Geometry: final body of the model. Coordinates: model frame, mm. A direction names the side the tool comes from. Round coordinates to 2 decimals unless told otherwise and drop trailing zeros. Order: outer loops, then holes, each group sorted by start corner. A loop starts at its lowest first (then second) coordinate and runs counter-clockwise, first axis right, second up. Notation, with made-up numbers: (20, 19) - (32, 19) arc R9 cw to (32, 36) - close; hole circle Ø7 at (2.25, 20). An arc over 180 degrees is marked (long way). Put each result on its own line as item: value. Start each with the question number.
(1) Access query for faces 3 (the face through (22.121, 0.986, -7.114)), 4 (the face through (-17.948, 0.986, 9.927)), 5 (the face through (5.273, 0.986, 18.594)). Directions: +Z, -Z, +X, -X, +Y, -Y. A direction counts if a zero-diameter tool reaches every point of the face in a straight line with its end or side. Return the directions, or none.
(2) Pull-direction query (Z, two-part tool) for faces 1 (the face through (22.596, 0.986, -2.222)), 2 (the face through (17.22, 0.99, 15.6)); classes: released by +Z, released by -Z, zero draft, split by the parting line, or undercut.
(3) Section A-A (x = 0). Output: boundary loops of the cut face in (y, z), and give its area (3 significant figures).
(4) Pin query (flat end, axial travel): P1, Ø0.6, axis at x = -5, y = 1, coming from the +Z side; P2, Ø1, axis at x = 4, y = 1, coming from the -Z side; P3, Ø0.6, axis at y = 1, z = 5.5, coming from the +X side. Return the tip coordinate at first contact, or that it passes through.
(5) Section B-B (z = 0). Output: boundary loops of the cut face in (x, y), and give its area (3 significant figures).
(6) Material intervals for L1, parallel to X at y = 0.45, z = 7.5; L2, parallel to X at y = 1.75, z = -21; L3, parallel to Z at x = 5.5, y = 1.35, sorted ascending. Write a range as [from, to].
(7) Section C-C (y = 0.45). Count the separate pieces of the cut face and the enclosed holes in it, and give its area (3 significant figures).
from build123d import *

# Parameters (mm, degrees)
SKETCH_1_R      = 1
SKETCH_1_R_2    = 12.835097572
EXTRUDE_1_DEPTH = 2


with BuildPart() as part:
    # 草图1 → 凸台-拉伸1 (new body)
    with BuildSketch(Plane(origin=(0, 0, 0), x_dir=(1, 0, 0), z_dir=(0, 1, 0))):
        with BuildLine():
            Line((7.150459564, 22.71458211), (2.584896164, 22.71458211))
            Line((2.584896164, 22.71458211), (-1.893440977, 18.236244969))
            Line((-1.893440977, 18.236244969), (-6.310791907, 15.68588622))
            ThreePointArc((-6.310791907, 15.68588622), (-7.676817311, 16.051911624), (-7.310791907, 17.417937028))
            Line((-7.310791907, 17.417937028), (-3.177406319, 19.80434831))
            ThreePointArc((-3.177406319, 19.80434831), (-2.244981501, 22.637541774), (-5.164811424, 23.246634926))
            Line((-5.164811424, 23.246634926), (-9.118705311, 20.963853226))
            Line((-9.118705311, 20.963853226), (-10.757890471, 14.846330924))
            Line((-10.757890471, 14.846330924), (-13.30824922, 10.428979994))
            ThreePointArc((-13.30824922, 10.428979994), (-14.674274623, 10.06295459), (-15.040300027, 11.428979994))
            Line((-15.040300027, 11.428979994), (-12.653888745, 15.562365582))
            ThreePointArc((-12.653888745, 15.562365582), (-13.262981897, 18.482195505), (-16.096175362, 17.549770686))
            Line((-16.096175362, 17.549770686), (-18.378957062, 13.5958768))
            Line((-18.378957062, 13.5958768), (-16.739771901, 7.478354497))
            Line((-16.739771901, 7.478354497), (-16.739771901, 2.377637001))
            ThreePointArc((-16.739771901, 2.377637001), (-17.739771901, 1.377637001), (-18.739771901, 2.377637001))
            Line((-18.739771901, 2.377637001), (-18.739771901, 7.150459564))
            ThreePointArc((-18.739771901, 7.150459564), (-20.727177006, 9.374559877), (-22.71458211, 7.150459564))
            Line((-22.71458211, 7.150459564), (-22.71458211, 2.584896164))
            Line((-22.71458211, 2.584896164), (-18.236244969, -1.893440977))
            Line((-18.236244969, -1.893440977), (-15.68588622, -6.310791907))
            ThreePointArc((-15.68588622, -6.310791907), (-16.051911624, -7.676817311), (-17.417937028, -7.310791907))
            Line((-17.417937028, -7.310791907), (-19.80434831, -3.177406319))
            ThreePointArc((-19.80434831, -3.177406319), (-22.637541774, -2.244981501), (-23.246634926, -5.164811424))
            Line((-23.246634926, -5.164811424), (-20.963853226, -9.118705311))
            Line((-20.963853226, -9.118705311), (-14.846330924, -10.757890471))
            Line((-14.846330924, -10.757890471), (-10.428979994, -13.30824922))
            ThreePointArc((-10.428979994, -13.30824922), (-10.06295459, -14.674274623), (-11.428979994, -15.040300027))
            Line((-11.428979994, -15.040300027), (-15.562365582, -12.653888745))
            ThreePointArc((-15.562365582, -12.653888745), (-18.482195505, -13.262981897), (-17.549770686, -16.096175362))
            Line((-17.549770686, -16.096175362), (-13.5958768, -18.378957062))
            Line((-13.5958768, -18.378957062), (-7.478354497, -16.739771901))
            Line((-7.478354497, -16.739771901), (-2.377637001, -16.739771901))
            ThreePointArc((-2.377637001, -16.739771901), (-1.377637001, -17.739771901), (-2.377637001, -18.739771901))
            Line((-2.377637001, -18.739771901), (-7.150459564, -18.739771901))
            ThreePointArc((-7.150459564, -18.739771901), (-9.374559877, -20.727177006), (-7.150459564, -22.71458211))
            Line((-7.150459564, -22.71458211), (-2.584896164, -22.71458211))
            Line((-2.584896164, -22.71458211), (1.893440977, -18.236244969))
            Line((1.893440977, -18.236244969), (6.310791907, -15.68588622))
            ThreePointArc((6.310791907, -15.68588622), (7.676817311, -16.051911624), (7.310791907, -17.417937028))
            Line((7.310791907, -17.417937028), (3.177406319, -19.80434831))
            ThreePointArc((3.177406319, -19.80434831), (2.244981501, -22.637541774), (5.164811424, -23.246634926))
            Line((5.164811424, -23.246634926), (9.118705311, -20.963853226))
            Line((9.118705311, -20.963853226), (10.757890471, -14.846330924))
            Line((10.757890471, -14.846330924), (13.30824922, -10.428979994))
            ThreePointArc((13.30824922, -10.428979994), (14.674274623, -10.06295459), (15.040300027, -11.428979994))
            Line((15.040300027, -11.428979994), (12.653888745, -15.562365582))
            ThreePointArc((12.653888745, -15.562365582), (13.262981897, -18.482195505), (16.096175362, -17.549770686))
            Line((16.096175362, -17.549770686), (18.378957062, -13.5958768))
            Line((18.378957062, -13.5958768), (16.739771901, -7.478354497))
            Line((16.739771901, -7.478354497), (16.739771901, -2.377637001))
            ThreePointArc((16.739771901, -2.377637001), (17.739771901, -1.377637001), (18.739771901, -2.377637001))
            Line((18.739771901, -2.377637001), (18.739771901, -7.150459564))
            ThreePointArc((18.739771901, -7.150459564), (20.727177006, -9.374559877), (22.71458211, -7.150459564))
            Line((22.71458211, -7.150459564), (22.71458211, -2.584896164))
            Line((22.71458211, -2.584896164), (18.236244969, 1.893440977))
            Line((18.236244969, 1.893440977), (15.68588622, 6.310791907))
            ThreePointArc((15.68588622, 6.310791907), (16.051911624, 7.676817311), (17.417937028, 7.310791907))
            Line((17.417937028, 7.310791907), (19.80434831, 3.177406319))
            ThreePointArc((19.80434831, 3.177406319), (22.637541774, 2.244981501), (23.246634926, 5.164811424))
            Line((23.246634926, 5.164811424), (20.963853226, 9.118705311))
            Line((20.963853226, 9.118705311), (14.846330924, 10.757890471))
            Line((14.846330924, 10.757890471), (10.428979994, 13.30824922))
            ThreePointArc((10.428979994, 13.30824922), (10.06295459, 14.674274623), (11.428979994, 15.040300027))
            Line((11.428979994, 15.040300027), (15.562365582, 12.653888745))
            ThreePointArc((15.562365582, 12.653888745), (18.482195505, 13.262981897), (17.549770686, 16.096175362))
            Line((17.549770686, 16.096175362), (13.5958768, 18.378957062))
            Line((13.5958768, 18.378957062), (7.478354497, 16.739771901))
            Line((7.478354497, 16.739771901), (2.377637001, 16.739771901))
            ThreePointArc((2.377637001, 16.739771901), (1.377637001, 17.739771901), (2.377637001, 18.739771901))
            Line((2.377637001, 18.739771901), (7.150459564, 18.739771901))
            ThreePointArc((7.150459564, 18.739771901), (9.374559877, 20.727177006), (7.150459564, 22.71458211))
        make_face()
        with Locations(Location((7.374559877, 20.727177006, 0), (0, 0, 270))):
            Circle(SKETCH_1_R, mode=Mode.SUBTRACT)
        with Locations(Location((16.750144698, 14.262981897, 0), (0, 0, 270))):
            Circle(SKETCH_1_R, mode=Mode.SUBTRACT)
        with Locations(Location((21.637541774, 3.977032308, 0), (0, 0, 270))):
            Circle(SKETCH_1_R, mode=Mode.SUBTRACT)
        with Locations(Location((20.727177006, -7.374559877, 0), (0, 0, 270))):
            Circle(SKETCH_1_R, mode=Mode.SUBTRACT)
        with Locations(Location((14.262981897, -16.750144698, 0), (0, 0, 270))):
            Circle(SKETCH_1_R, mode=Mode.SUBTRACT)
        with Locations(Location((3.977032308, -21.637541774, 0), (0, 0, 270))):
            Circle(SKETCH_1_R, mode=Mode.SUBTRACT)
        with Locations(Location((-7.374559877, -20.727177006, 0), (0, 0, 270))):
            Circle(SKETCH_1_R, mode=Mode.SUBTRACT)
        with Locations(Location((-16.750144698, -14.262981897, 0), (0, 0, 270))):
            Circle(SKETCH_1_R, mode=Mode.SUBTRACT)
        with Locations(Location((-21.637541774, -3.977032308, 0), (0, 0, 270))):
            Circle(SKETCH_1_R, mode=Mode.SUBTRACT)
        with Locations(Location((-20.727177006, 7.374559877, 0), (0, 0, 270))):
            Circle(SKETCH_1_R, mode=Mode.SUBTRACT)
        with Locations(Location((-14.262981897, 16.750144698, 0), (0, 0, 270))):
            Circle(SKETCH_1_R, mode=Mode.SUBTRACT)
        with Locations(Location((-3.977032308, 21.637541774, 0), (0, 0, 270))):
            Circle(SKETCH_1_R, mode=Mode.SUBTRACT)
        with Locations(Location((0, 0, 0), (0, 0, 270))):
            Circle(SKETCH_1_R_2, mode=Mode.SUBTRACT)
    extrude(amount=EXTRUDE_1_DEPTH)


solid = part.part
Checks:
1. face 3: -Z, +X, +Y, -Y
1. face 4: -X, +Y, -Y
1. face 5: +Y, -Y
2. face 1: undercut
2. face 2: released by +Z
3. outline: (0, -20.13) - (2, -20.13) - (2, -12.84) - (0, -12.84) - close; (0, 12.84) - (2, 12.84) - (2, 20.13) - (0, 20.13) - close
3. area: 29.2 mm²
4. P1: stops at z = 22.71
4. P2: stops at z = -22.71
4. P3: stops at x = 22.71
5. outline: (-20.13, 0) - (-12.84, 0) - (-12.84, 2) - (-20.13, 2) - close; (12.84, 0) - (20.13, 0) - (20.13, 2) - (12.84, 2) - close
5. area: 29.2 mm²
6. L1: x = [-21.9, -17.28], [-15.83, -10.42], [10.42, 16.75], [18.73, 19.74], [21.72, 22.72]
6. L2: x = [-9.06, -4.75], [-3.21, -2.08], [0.87, 6.41], [8.34, 9.36]
6. L3: z = [-22.71, -18.74], [-16.74, -11.6], [11.6, 16.15], [18.46, 23.05]
7. separate pieces: 1
7. enclosed holes: 13
7. area: 850 mm²
